Check sheet for the modelled part. Datum: model origin and axes. Units: mm. Coordinates: 2 decimals unless noted, no trailing zeros. Write each loop counter-clockwise with the first axis right and the second up, starting at its lowest first coordinate (ties: lowest second). Pieces come first, ordered by that corner, then holes. Notation, with made-up numbers: (16.5, -11.75) - (26.5, -11.75) arc R23 ccw to (26.5, 0.25) - close; hole circle Ø7 at (80, 81.5). An arc over 180 degrees is marked (long way). Answer as CSV lines item,"result". Start each with the question number.
from build123d import *

# Parameters (mm, degrees)
ESQUISSE1_R                  = 55
BOSS_EXTRU_1_DEPTH           = 15
TROU_TARAUD_M101_D           = 8.5
R_P_TITION_CIRCULAIRE1_COUNT = 6
ESQUISSE4_R                  = 39
ENL_V_MAT_EXTRU_1_DEPTH      = 16


with BuildPart() as part:
    # Esquisse1 → Boss.-Extru.1 (new body)
    with BuildSketch(Plane.XY):
        Circle(ESQUISSE1_R)
    extrude(amount=BOSS_EXTRU_1_DEPTH)

    # Trou taraudé M101 (through all)
    with Locations(Plane.XY.offset(15)):
        with Locations((0, 47)):
            trou_taraud_m101 = Hole(TROU_TARAUD_M101_D / 2)

    # Répétition circulaire1: Trou taraudé M101 ×6 about axis
    r_p_tition_circulaire1_axis = Axis((0, 0, 0), (0, 0, 1))
    for i in range(1, R_P_TITION_CIRCULAIRE1_COUNT):
        add(trou_taraud_m101.rotate(r_p_tition_circulaire1_axis, i * 360 / R_P_TITION_CIRCULAIRE1_COUNT), mode=Mode.SUBTRACT)

    # Esquisse4 → Enlèv. mat.-Extru.1 (cut, through all)
    with BuildSketch(Plane.XY.offset(15)):
        Circle(ESQUISSE4_R)
    extrude(amount=-ENL_V_MAT_EXTRU_1_DEPTH, mode=Mode.SUBTRACT)


solid = part.part
(1) Material ranges on probe 1 along Y at (x, z) = (0, 11.75); probe 2 along Y at (x, z) = (40.5, 6); probe 3 along Y at (x, z) = (-35.5, 2), recorded low to high. Write a range as from..to.
(2) Release check for a two-part mould opening along X. For faces 1 (the face through (-5.077, 38.668, 7.605)), 2 (the face through (-11.923, -53.692, 7.395)), 3 (the face through (16, -36, 15)) record: pulls with the +X half, pulls with the -X half, needs draft (parallel to the pull), parting line crosses it, or undercut.
(3) Go/stop test with flat-tipped pins: P1, Ø8, axis at x = -12, z = 8.5, coming from the -Y side; P2, Ø6, axis at y = 23.5, z = 10, coming from the -X side; P3, Ø8, axis at x = -28, z = 8, coming from the +Y side; P4, Ø4, axis at x = -24.5, y = -26, coming from the +Z side. Record where each tip stops, or that it passes through.
(4) Cross-section at D-D on z = 9.25. Record the boundary of the cut face in (x, y).
(5) Cross-section at B-B on x = 0. Record the boundary of the cut face in (y, z).
(6) Cross-section at C-C on x = -31. Record the boundary of the cut face in (y, z), plus the area to 3 significant figures.
(7) Cross-section at A-A on y = 0. Record the boundary of the cut face in (x, z).
Checked values:
1,probe 1,"-55..-51.25, -42.75..-39, 39..42.75, 51.25..55"
1,probe 2,"-37.21..-27.75, -19.25..19.25, 27.75..37.21"
1,probe 3,"-42.01..-16.15, 16.15..42.01"
2,face 1,"undercut"
2,face 2,"parting line crosses it"
2,face 3,"needs draft"
3,P1,"y = -54.42"
3,P2,"x = -51.04"
3,P3,"y = 49.49"
3,P4,"through"
4,outline,"circle Ø110 at (0, 0); hole circle Ø8.5 at (-40.7, -23.5); hole circle Ø8.5 at (-40.7, 23.5); hole circle Ø78 at (0, 0); hole circle Ø8.5 at (0, -47); hole circle Ø8.5 at (0, 47); hole circle Ø8.5 at (40.7, -23.5); hole circle Ø8.5 at (40.7, 23.5)"
5,outline,"(-55, 0) - (-51.25, 0) - (-51.25, 15) - (-55, 15) - close; (-42.75, 0) - (-39, 0) - (-39, 15) - (-42.75, 15) - close; (39, 0) - (42.75, 0) - (42.75, 15) - (39, 15) - close; (51.25, 0) - (55, 0) - (55, 15) - (51.25, 15) - close"
6,outline,"(-45.43, 0) - (-23.66, 0) - (-23.66, 15) - (-45.43, 15) - close; (23.66, 0) - (45.43, 0) - (45.43, 15) - (23.66, 15) - close"
6,area,"653 mm^2"
7,outline,"(-55, 0) - (-39, 0) - (-39, 15) - (-55, 15) - close; (39, 0) - (55, 0) - (55, 15) - (39, 15) - close"
